Design review of the part built by this model. Coordinates are the model's own, in mm. A direction names the side the tool comes from. Round coordinates to 2 decimals unless told otherwise and drop trailing zeros. Loops run counter-clockwise (first coordinate to the right, second up) from the corner with the lowest first, then second, coordinate; pieces in that order, holes last. Notation, with made-up numbers: (8, 3) - (12, 3) arc R22 cw to (12, 29) - close; hole circle Ø5 at (-12, -38). An arc over 180 degrees is marked (long way). One line per question, with ' | ' between items. Start each with the question number.
from build123d import *

# Parameters (mm, degrees)
SKETCH1_R                     = 31.5
EXTRUDE1_DEPTH                = 4
SKETCH3_R                     = 9
EXTRUDE2_DEPTH                = 6
M11_0_11_DIAMETER_HOLE1_D     = 11
M11_0_11_DIAMETER_HOLE1_DEPTH = 10
M11_0_11_DIAMETER_HOLE1_TIP   = 3.304733405
EXTRUDE4_DEPTH                = 13
CIRPATTERN2_COUNT             = 6
SKETCH7_R                     = 9
SKETCH7_R_2                   = 8.1
EXTRUDE5_DEPTH                = 17


with BuildPart() as part:
    # Sketch1 → Extrude1 (new body)
    with BuildSketch(Plane.XY):
        Circle(SKETCH1_R)
    extrude(amount=EXTRUDE1_DEPTH)

    # Sketch3 → Extrude2 (add)
    with BuildSketch(Plane.XY.offset(4)):
        Circle(SKETCH3_R)
    extrude(amount=EXTRUDE2_DEPTH)

    # M11.0 _11_ Diameter Hole1
    with Locations(Plane.XY.offset(10)):
        with Locations((0, 0)):
            Hole(M11_0_11_DIAMETER_HOLE1_D / 2, depth=M11_0_11_DIAMETER_HOLE1_DEPTH)
            with Locations((0, 0, -(M11_0_11_DIAMETER_HOLE1_DEPTH + M11_0_11_DIAMETER_HOLE1_TIP / 2))):  # 118° drill point
                Cone(0, M11_0_11_DIAMETER_HOLE1_D / 2, M11_0_11_DIAMETER_HOLE1_TIP, mode=Mode.SUBTRACT)

    # Sketch2_8 → Extrude4 (add)
    with BuildSketch(Plane.XY.offset(4)):
        with BuildLine():
            ThreePointArc((-9.844910533, 0.62593686), (-18.139880625, -12.361871339), (-15.335083755, -27.515181378))
            ThreePointArc((-15.335083755, -27.515181378), (-13.401012303, -28.5072424), (-11.403128973, -29.363559894))
            ThreePointArc((-11.403128973, -29.363559894), (-16.511325203, -17.190045629), (-12.454740571, -4.626915468))
            ThreePointArc((-12.454740571, -4.626915468), (-9.953426801, -3.486629519), (-7.573470906, -4.862359348))
            ThreePointArc((-7.573470906, -4.862359348), (-8.889824652, -1.403929362), (-8.703301392, 2.291843117))
            ThreePointArc((-8.703301392, 2.291843117), (-9.129712004, 1.359939965), (-9.844910533, 0.62593686))
        make_face()
    extrude4 = extrude(amount=EXTRUDE4_DEPTH)

    # CirPattern2: Extrude4 ×6 about axis
    cirpattern2_axis = Axis((0, 0, 0), (0, 0, 1))
    for i in range(1, CIRPATTERN2_COUNT):
        add(extrude4.rotate(cirpattern2_axis, i * 360 / CIRPATTERN2_COUNT))

    # Sketch7 → Extrude5 (add)
    with BuildSketch(Plane(origin=(0, 0, 0), x_dir=(-1, 0, 0), z_dir=(0, 0, -1))):
        Circle(SKETCH7_R)
        with Locations(Location((0, 0, 0), (0, 0, 180))):  # turned: the seam where the file's is
            Circle(SKETCH7_R_2, mode=Mode.SUBTRACT)
    extrude(amount=-EXTRUDE5_DEPTH)


solid = part.part
1. Machinability: for faces 3 (the face through (-1.756, 7.907, 13.451)), 4 (the face through (6.99, 5.67, 10.41)), which of the approach directions +Z, -Z, +X, -X, +Y, -Y give a long, thin tool a straight path to every point of the face, cutting with its end or side? Answer none if there is none.
2. Take a section at B-B, the plane x = -21. Give the boundary of the cut face in (y, z).
3. To check wall thickness, follow line 1 along Y through (x, z) = (0, 14.75); line 2 along X through (y, z) = (-1, 15.5); line 3 along Y through (x, z) = (0, 6). State the ranges of each line that lie inside material, in increasing order.
4. The part is to be moulded in two halves that separate along X. For faces 1 (the face through (7, 0, 0)), 2 (the face through (1.98, 10.4, 10.41)), say which applies: pulls with the +X half, pulls with the -X half, needs draft (parallel to the pull), parting line crosses it, or undercut.
5. Take a section at A-A, the plane z = 1.5. Give the boundary of the cut face in (x, y).
6. Clearance check with flat-ended pins moving along their axes: P1, Ø1, axis at x = -20.5, z = 2.5, coming from the -Y side; P2, Ø7.5, axis at x = -7, y = 17.5, coming from the +Z side; P3, Ø8, axis at x = -1, y = -2.5, coming from the +Z side. State where each tip first meets the part, or that it passes through.
7. Take a section at C-C, the plane y = 16. Give the boundary of the cut face in (x, z), then the cut area to 3 significant figures.
8. Take a section at D-D, the plane y = -19.5. Give the boundary of the cut face in (x, z), then the cut area to 3 significant figures.
Answer list:
1) face 3: +Z | face 4: +Z, +Y
2) outline: (-23.48, 0) - (23.48, 0) - (23.48, 4) - (9.06, 4) - (9.06, 17) - (6.88, 17) - (6.88, 4) - (-23.48, 4) - close
3) line 1: y = -20.3 to -17.15, -9.04 to -8.1, 8.1 to 9.04, 17.15 to 20.3 | line 2: x = -31.48 to -29.5, -11.82 to -8.04, 8.04 to 9.42, 28.2 to 30.63 | line 3: y = -20.3 to -17.15, -9.04 to -5.5, 5.5 to 9.04, 17.15 to 20.3
4) face 1: needs draft | face 2: undercut
5) outline: circle Ø63 at (0, 0); hole circle Ø11 at (0, 0)
6) P1: stops at y = -24.34 | P2: stops at z = 4 | P3: stops at z = 10
7) outline: (-27.13, 0) - (27.13, 0) - (27.13, 4) - (18.52, 4) - (18.52, 17) - (16.52, 17) - (16.52, 4) - (3.07, 4) - (3.07, 17) - (0.76, 17) - (0.76, 4) - (-27.13, 4) - close | area: 273 mm²
8) outline: (-24.74, 0) - (24.74, 0) - (24.74, 4) - (2, 4) - (2, 17) - (-0.7, 17) - (-0.7, 4) - (-16.27, 4) - (-16.27, 17) - (-18.3, 17) - (-18.3, 4) - (-24.74, 4) - close | area: 259 mm²
